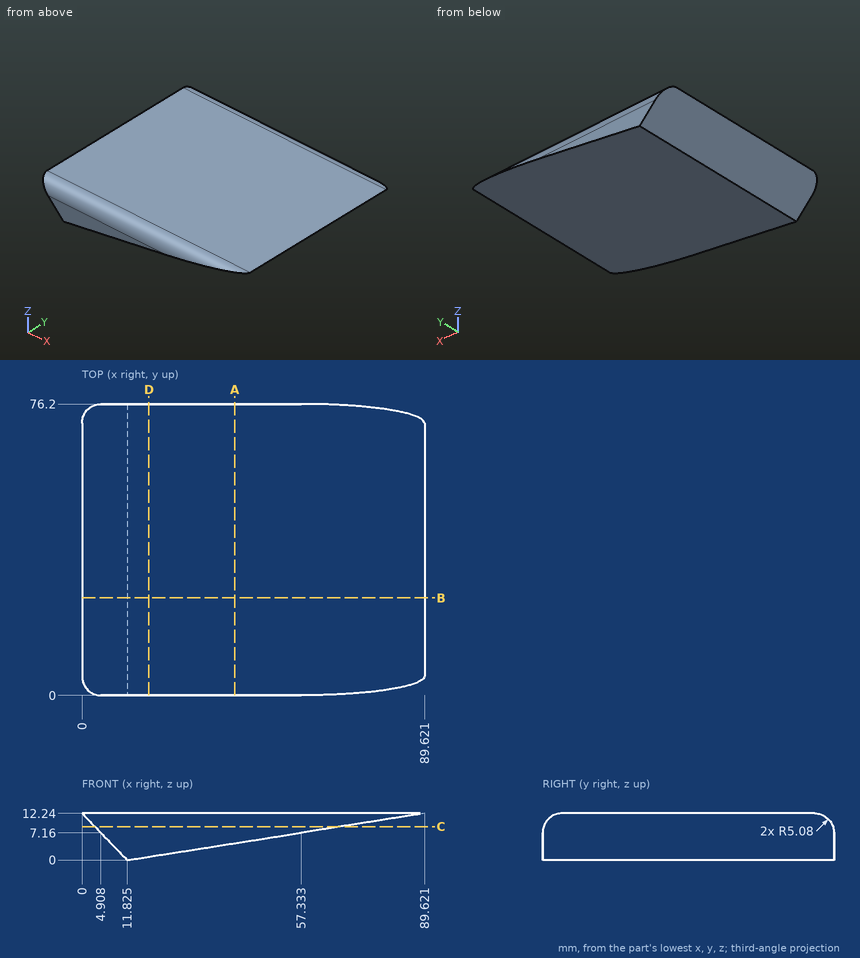
Job drawing, mm, ordinate dimensions from the low corner. One solid piece. Coordinates: 2 decimals unless noted, no trailing zeros. Write each loop counter-clockwise with the first axis right and the second up, starting at its lowest first coordinate (ties: lowest second). Pieces come first, ordered by that corner, then holes.
Item 1: Slice it at B-B (y = 25.5). Write the cut outline in (x, z) (1 decimal).
Item 2: Slice it at C-C (z = 8.75). Write the cut outline in (x, y) (1 decimal).
Item 3: Probe line 1 (Z direction, x = 18.5, y = 49); line 2 (Z direction, x = 5.5, y = 64) (1 decimal); line 3 (Y direction, x = 55, z = 9.5). List the from-to ranges inside material, lowest first.
Item 4: Pin check, flat tips, straight feed: pin 1 (1.5 mm diameter, centred on x = 59, y = 29.5, fed in from -Z); pin 2 (4 mm diameter, centred on y = 58.5, z = 7, fed in from -X); pin 3 (5 mm diameter, centred on x = 36.5, z = 1.5, fed in from +Y); pin 4 (6 mm diameter, centred on x = 72, y = 36.5, fed in from -Z) (1 decimal). Stop position of each tip, or through.
Item 5: Slice it at A-A (x = 40). Write the cut outline in (y, z), and give its area (3 significant figures).
Item 6: Slice it at D-D (x = 17.5). Write the cut outline in (y, z).
Results found:
1. outline: (0, 12.2) - (11.8, 0) - (89.6, 12.2) - close
2. outline: (3.4, 0.3) - (67.4, 0.3) - (67.4, 75.9) - (3.4, 75.9) - close
3. line 1: z = 1.05 to 12.24
3. line 2: z = 6.5 to 12.2
3. line 3: y = 0.57 to 75.63
4. pin 1: stops at z = 7.3
4. pin 2: stops at x = 3.13
4. pin 3: stops at y = 76.2
4. pin 4: stops at z = 9
5. outline: (0, 4.43) - (76.2, 4.43) - (76.2, 7.16) arc R5.08 ccw to (71.12, 12.24) - (5.08, 12.24) arc R5.08 ccw to (0, 7.16) - close
5. area: 584 mm2
6. outline: (0, 0.89) - (76.2, 0.89) - (76.2, 7.16) arc R5.08 ccw to (71.12, 12.24) - (5.08, 12.24) arc R5.08 ccw to (0, 7.16) - close
